```python
from build123d import *

# Parameters (mm, degrees)
SKETCH1_W               = 250
SKETCH1_H               = 7
SKETCH2_W               = 68
SKETCH2_H               = 7
BOSS_EXTRUDE1_DEPTH     = 25
SKETCH3_W               = 4
SKETCH3_H               = 7.5
BOSS_EXTRUDE2_DEPTH     = 15
FILLET1_R               = 3.5
SKETCH5_R               = 2.5
SKETCH5_W               = 4
SKETCH5_H               = 14
BOSS_EXTRUDE3_DEPTH     = 30
FILLET2_R               = 3.5
CUT_EXTRUDE1_DEPTH      = 195.461435879
CUT_EXTRUDE1_DEPTH_BACK = 195.461435879
SKETCH6_R               = 2
SKETCH4_R               = 2
CUT_EXTRUDE2_DEPTH      = 144.418966785
CUT_EXTRUDE3_START      = -15
SKETCH7_R               = 2.5
CUT_EXTRUDE3_DEPTH      = 15


with BuildPart() as part:
    # Sketch1 → Revolve-Thin1 (revolve)
    with BuildSketch(Plane.XY, mode=Mode.PRIVATE) as revolve_thin1_sk:
        with Locations((0, 3.5)):
            Rectangle(SKETCH1_W, SKETCH1_H)
    revolve(revolve_thin1_sk.sketch.rotate(Axis((-125, 0, 0), (1, 0, 0)), 180), axis=Axis((-125, 0, 0), (1, 0, 0)))

    # Sketch2 → Boss-Extrude1 (add)
    with BuildSketch(Plane(origin=(0, 0, 0), x_dir=(1, 0, 0), z_dir=(0, 1, 0))):
        Rectangle(SKETCH2_W, SKETCH2_H)
    extrude(amount=BOSS_EXTRUDE1_DEPTH)

    # Sketch3 → Boss-Extrude2 (add)
    with BuildSketch(Plane.XY.offset(3.5)):
        with Locations((-11, 21.25)):
            Rectangle(SKETCH3_W, SKETCH3_H)
        with Locations((0, 21.25)):
            Rectangle(SKETCH3_W, SKETCH3_H)
        with Locations((11, 21.25)):
            Rectangle(SKETCH3_W, SKETCH3_H)
    extrude(amount=BOSS_EXTRUDE2_DEPTH)

    # Fillet1
    fillet1_edges = [part.edges().sort_by_distance(p)[0] for p in [
        (-11, 17.5, 18.5),
        (-11, 25, 18.5),
        (0, 17.5, 18.5),
        (0, 25, 18.5),
        (11, 17.5, 18.5),
        (11, 25, 18.5),
    ]]
    fillet(fillet1_edges, radius=FILLET1_R)

    # Sketch5 → Boss-Extrude3 (add)
    with BuildSketch(Plane.XY):
        with Locations(Location((31, 4.5, 0), (0, 0, 141.327270593))):
            Circle(SKETCH5_R)
        with Locations((-52.5, 0)):
            Rectangle(SKETCH5_W, SKETCH5_H)
        with Locations((-63.5, 0)):
            Rectangle(SKETCH5_W, SKETCH5_H)
        with Locations((63.5, 0)):
            Rectangle(SKETCH5_W, SKETCH5_H)
        with Locations((52.5, 0)):
            Rectangle(SKETCH5_W, SKETCH5_H)
    extrude(amount=BOSS_EXTRUDE3_DEPTH)

    # Fillet2
    fillet2_edges = [part.edges().sort_by_distance(p)[0] for p in [
        (-63.5, 7, 30),
        (-63.5, -7, 30),
        (63.5, 7, 30),
        (63.5, -7, 30),
        (52.5, 7, 30),
        (52.5, -7, 30),
        (-52.5, -7, 30),
        (-52.5, 7, 30),
    ]]
    fillet(fillet2_edges, radius=FILLET2_R)

    # Sketch6 → Cut-Extrude1 (cut, two sides: drawn at the far end of the back side and taken through both)
    with BuildSketch(Plane.ZY.offset(65.5).offset(-CUT_EXTRUDE1_DEPTH_BACK)):
        with Locations(Location((24, 3, 0), (0, 0, 180))):
            Circle(SKETCH6_R)
        with Locations(Location((24, -3, 0), (0, 0, 180))):
            Circle(SKETCH6_R)
    extrude(amount=CUT_EXTRUDE1_DEPTH + CUT_EXTRUDE1_DEPTH_BACK, mode=Mode.SUBTRACT)

    # Sketch4 → Cut-Extrude2 (cut, through all)
    with BuildSketch(Plane.ZY.offset(13)):
        with Locations(Location((12, 21, 0), (0, 0, 270))):
            Circle(SKETCH4_R)
    extrude(amount=-CUT_EXTRUDE2_DEPTH, mode=Mode.SUBTRACT)

    # Sketch7 → Cut-Extrude3 (cut)
    with BuildSketch(Plane.XY.offset(30).offset(CUT_EXTRUDE3_START)):
        with Locations(Location((31, 4.5, 0), (0, 0, 141.327270593))):
            Circle(SKETCH7_R)
    extrude(amount=CUT_EXTRUDE3_DEPTH, mode=Mode.SUBTRACT)


solid = part.part
```
Can you work these out from the model? Positions are in its coordinate system, mm. A direction names the side the tool comes from. Coordinates: 2 decimals unless noted, no trailing zeros. Loops run counter-clockwise (first coordinate to the right, second up) from the corner with the lowest first, then second, coordinate; pieces in that order, holes last. Notation, with made-up numbers: M 20.25,26 L 38.25,26 A28 cw 38.25,63 Z; hole C 4.25,81.25 d5. An arc over 180 degrees is marked long. Put each result on its own line as item: value. Start each with the question number.
(1) We'd pull the mould along Y, two halves only. Please class faces 4 (the face through (11, 17.5, 9)), 5 (the face through (0, 25, 2)), 6 (the face through (54.5, 0, 18)): +Y half, -Y half, draft (parallel to the pull), parting line (faces both ways), or undercut.
(2) Will these pins go through, and if not, where does the flat tip stop? pin 1 Ø3 at (x, z) = (11.5, 12) entering from -Y; pin 2 Ø3.5 at (y, z) = (3, 24) entering from -X; pin 3 Ø2 at (y, z) = (15.5, 0.5) entering from +X; pin 4 Ø4 at (y, z) = (21.5, 9) entering from -X.
(3) Imagine slicing it at A-A on x = 105.5. List the corners of the cut face in (y, z) for me.
(4) I need wall thicknesses on probe 1 along Y at (x, z) = (51.75, 24); probe 2 along X at (y, z) = (-0.5, 24); probe 3 along X at (y, z) = (6, 12). Which ranges of each line are inside material? Lowest first, please.
(5) Imagine slicing it at B-B on x = -31.5. List the corners of the cut face in (y, z) for me.
(6) Which directions (+Z, -Z, +X, -X, +Y, -Y) give clear straight access to the entire face, cutting with the end or side of a thin tool? Please do faces 1 (the face through (0, 15, -3.5)), 2 (the face through (13, 21, 9)), 3 (the face through (9, 21, 9)).
Worked answers:
1. face 4: undercut
1. face 5: +Y half
1. face 6: draft
2. pin 1: stops at y = 17.5
2. pin 2: passes through
2. pin 3: stops at x = 34
2. pin 4: stops at x = -13
3. outline: C 0,0 d14
4. probe 1: y = -7 to -5, -1 to 1, 5 to 7
4. probe 2: x = -65.5 to -61.5, -54.5 to -50.5, 50.5 to 54.5, 61.5 to 65.5
4. probe 3: x = -65.5 to -61.5, -54.5 to -50.5, 29 to 33, 50.5 to 54.5, 61.5 to 65.5
5. outline: M 6.06,-3.5 L 25,-3.5 L 25,3.5 L 6.06,3.5 A7 ccw long Z
6. face 1: -Z, +X, -X, +Y
6. face 2: +Z, +X, +Y
6. face 3: +Z, +Y
